Part model, mm, in its own coordinate system. A direction names the side the tool comes from. Round coordinates to 2 decimals unless told otherwise and drop trailing zeros. Write each loop counter-clockwise with the first axis right and the second up, starting at its lowest first coordinate (ties: lowest second). Pieces come first, ordered by that corner, then holes. Notation, with made-up numbers: M 58.25,86 L 117.25,86 A21 ccw 117.25,90 Z; hole C -27,-23 d11. An arc over 180 degrees is marked long. Answer as a JSON object with one key per item and string values. Group by question number.
1. Two-plate mould, pull along X, no slides. Class faces 3 (the face through (33.166, 4.452, 1.479)), 4 (the face through (10, 5, 1)), 5 (the face through (50.748, 6.415, 1.479)), 6 (the face through (-1.5, 0.07, 1.48)): +X half, -X half, draft (parallel to the pull), parting line (faces both ways), or undercut.
2. Drill centre lines: line 1 (Y direction, x = 0, z = 2.4); line 2 (X direction, y = -1.25, z = 0.3); line 3 (X direction, y = -0.25, z = 2.6). Where is each one in solid material? Low to high. Write a range as from..to.
3. Which spindle directions (+Z, -Z, +X, -X, +Y, -Y) get a long thin tool onto all of the face, cutting with end or side? Do faces 1 (the face through (33.414, 10.495, 1.479)), 2 (the face through (42.99, 5.85, 1.48)). Say none if no direction does.
4. Band-saw the part on C-C, the plane x = 19.5. Write the cut outline in (y, z).
5. Band-saw the part on A-A, the plane z = 1. Write the cut outline in (x, y), plus the area to 3 significant figures.
6. Band-saw the part on D-D, the plane x = 43.5. Write the cut outline in (y, z).
7. Drop a flat-ended pin along its axis: pin 1 (1.5 mm diameter, centred on x = 8, z = 1, fed in from +Y). Give the stop position or say it passes through.
8. Band-saw the part on B-B, the plane y = 0. Write the cut outline in (x, z), plus the area to 3 significant figures.
from build123d import *

# Parameters (mm, degrees)
SKETCH_1_R      = 1.5
EXTRUDE_1_DEPTH = 3


with BuildPart() as part:
    # 草图1 → 凸台-拉伸1 (new body)
    with BuildSketch(Plane.XY):
        with BuildLine():
            Line((20.05, 5), (0, 5))
            ThreePointArc((0, 5), (-5, 0), (0, -5))
            Line((0, -5), (22, -5))
            Line((22, -5), (26.644435765, 1.851814361))
            Line((26.644435765, 1.851814361), (39.871788822, 7.125781662))
            Line((39.871788822, 7.125781662), (46.188488025, 4.540007042))
            Line((46.188488025, 4.540007042), (55.437270307, 8.34264117))
            Line((55.437270307, 8.34264117), (53.72608495, 12.504593197))
            Line((53.72608495, 12.504593197), (46.409029503, 15.837507263))
            Line((46.409029503, 15.837507263), (20.05, 5))
        make_face()
        Circle(SKETCH_1_R, mode=Mode.SUBTRACT)
        with Locations((22, 0)):
            Circle(SKETCH_1_R, mode=Mode.SUBTRACT)
    extrude(amount=EXTRUDE_1_DEPTH)


solid = part.part
Worked answers:
{
 "1": {"face 3": "undercut", "face 4": "draft", "face 5": "+X half", "face 6": "undercut"},
 "2": {"line 1": "y = -5..-1.5, 1.5..5", "line 2": "x = -4.84..-0.83, 0.83..21.17, 22.83..24.54", "line 3": "x = -4.99..-1.48, 1.48..20.52, 23.48..25.22"},
 "3": {"face 1": "+Z, -Z, -X, +Y", "face 2": "+Z, -Z, -Y"},
 "4": {"outline": "M -5,0 L 5,0 L 5,3 L -5,3 Z"},
 "5": {"outline": "M 0,-5 L 22,-5 L 26.64,1.85 L 39.87,7.13 L 46.19,4.54 L 55.44,8.34 L 53.73,12.5 L 46.41,15.84 L 20.05,5 L 0,5 A5 ccw Z; hole C 0,0 d3; hole C 22,0 d3", "area": "483 mm^2"},
 "6": {"outline": "M 5.64,0 L 14.64,0 L 14.64,3 L 5.64,3 Z"},
 "7": {"pin 1": "stops at y = 5"},
 "8": {"outline": "M -5,0 L -1.5,0 L -1.5,3 L -5,3 Z; M 1.5,0 L 20.5,0 L 20.5,3 L 1.5,3 Z; M 23.5,0 L 25.39,0 L 25.39,3 L 23.5,3 Z", "area": "73.2 mm^2"}
}
